from build123d import *

# Parameters (mm, degrees)
F1_DEPTH = 19.05
F2_R     = 1.5
F3_DEPTH = 12.7
F4_R     = 2.5
F5_DEPTH = 12.7


with BuildPart() as f1:
    # F0 (on Front) → F1 (new body)
    with BuildSketch(Plane.XZ):
        with BuildLine():
            Line((-43.747465, 0), (6.252535, 0))
            Line((6.252535, 0), (6.252535, 1.900001))
            Line((6.252535, 1.900001), (-43.747465, 1.900001))
            ThreePointArc((-43.747465, 1.900001), (-46.057163, 3.443292), (-45.515231, 6.167766))
            Line((-45.515231, 6.167766), (-27.837562, 23.845436))
            Line((-27.837562, 23.845436), (-29.181065, 25.188939))
            Line((-29.181065, 25.188939), (-46.858735, 7.51127))
            ThreePointArc((-46.858735, 7.51127), (-47.812535, 2.716193), (-43.747465, 0))
        make_face()
    extrude(amount=-F1_DEPTH)

    # F2 (on face) → F3 (cut)
    with BuildSketch(Plane(origin=(-27.185002, 0, 27.185002), x_dir=(0, -1, 0), z_dir=(-0.707107, 0, 0.707107))):
        with Locations((-7.5, -10.322859)):
            Circle(F2_R)
        with Locations((-11.55, -10.322859)):
            Circle(F2_R)
    extrude(amount=-F3_DEPTH, mode=Mode.SUBTRACT)

    # F4 (on face) → F5 (cut)
    with BuildSketch(Plane(origin=(0, 0, 0), x_dir=(1, 0, 0), z_dir=(0, 0, -1))):
        with BuildLine():
            Line((-5.372359, -7.282656), (-16.72876, -7.282656))
            ThreePointArc((-16.72876, -7.282656), (-18.690573, -10.030443), (-16.175304, -12.282656))
            Line((-16.175304, -12.282656), (-5.164585, -12.282656))
            ThreePointArc((-5.164585, -12.282656), (-3.70868, -9.717839), (-5.372359, -7.282656))
        make_face()
        with Locations((-25.747465, -9.375455)):
            Circle(F4_R)
    extrude(amount=-F5_DEPTH, mode=Mode.SUBTRACT)


solid = f1.part
Source: CAD feature listing. Evaluate the final solid. Frame: model axes, mm. A direction names the side the tool comes from. Round coordinates to 2 decimals unless told otherwise and drop trailing zeros. Loops run counter-clockwise (first coordinate to the right, second up) from the corner with the lowest first, then second, coordinate; pieces in that order, holes last. Notation, with made-up numbers: (-35.5, 62) - (-8.5, 62) arc R22 cw to (-8.5, 99) - close; hole circle Ø10 at (23, 74). An arc over 180 degrees is marked (long way). Write item = value, one per line. Start each with the question number.
(1) Section query D-D, the plane x = -42.5. Output: boundary loops of the cut face in (y, z).
(2) Ray query, line 1 along Z through (x, y) = (2.5, 5.25); line 2 along X through (y, z) = (10.5, 4.5); line 3 along Z through (x, y) = (-30.5, 3.5). Return the intervals inside material, ascending. Write a range as from..to.
(3) Pin query (flat end, axial travel): pin 1 (4 mm diameter, centred on y = 11.5, z = 14, fed in from +X); pin 2 (6 mm diameter, centred on y = 9.5, z = 15, fed in from -X); pin 3 (5 mm diameter, centred on y = 9, z = 10.5, fed in from +X). Return the tip coordinate at first contact, or that it passes through.
(4) Section query A-A, the plane x = -6. Output: boundary loops of the cut face in (y, z), plus the area to 3 significant figures.
(5) Pull-direction query (Z, two-part tool) for faces 1 (the face through (-3.707, 9.761, 0.937)), 2 (the face through (-46.041, 9.392, 3.405)), 3 (the face through (-19, 9, 0)); classes: +Z half, -Z half, draft (parallel to the pull), parting line (faces both ways), or undercut.
(6) Section query B-B, the plane y = 11.25. Output: boundary loops of the cut face in (x, z).
(7) Set-up query: faces 4 (the face through (-11, 12.283, 1)), 5 (the face through (-18, 7, 1.9)), 6 (the face through (-28.5, 9.39, 24.51)). Return all of +Z, -Z, +X, -X, +Y, -Y with unobstructed straight access to the full face (end or side cutting, diameter ignored); none if empty.
(8) Section query C-C, the plane y = 16.5. Output: boundary loops of the cut face in (x, z).
Conclusion:
q1.outline = (0, 0) - (19.05, 0) - (19.05, 1.9) - (0, 1.9) - close; (0, 9.18) - (19.05, 9.18) - (19.05, 11.87) - (0, 11.87) - close
q2.line_1 = 0..1.9
q2.line_2 = -48.15..-46.25
q2.line_3 = 0..1.9, 21.18..23.87
q3.pin_1 = -35.68
q3.pin_2 = -42.37
q3.pin_3 = -38.68
q4.outline = (0, 0) - (7.28, 0) - (7.28, 1.9) - (0, 1.9) - close; (12.28, 0) - (19.05, 0) - (19.05, 1.9) - (12.28, 1.9) - close
q4.area = 26.7 mm2
q5.face_1 = draft
q5.face_2 = undercut
q5.face_3 = -Z half
q6.outline = (-46.86, 7.51) arc R4.4 ccw to (-43.75, 0) - (-27.4, 0) - (-27.4, 1.9) - (-43.75, 1.9) arc R2.5 cw to (-45.52, 6.17) - (-34.18, 17.5) - (-35.52, 18.85) - close; (-33.45, 20.92) - (-32.1, 19.58) - (-27.84, 23.85) - (-29.18, 25.19) - close; (-24.09, 0) - (-18.21, 0) - (-18.21, 1.9) - (-24.09, 1.9) - close; (-4.09, 0) - (6.25, 0) - (6.25, 1.9) - (-4.09, 1.9) - close
q7.face_4 = +Z, -Z
q7.face_5 = +X, +Y, -Y
q7.face_6 = +Z, +X, +Y, -Y
q8.outline = (-46.86, 7.51) arc R4.4 ccw to (-43.75, 0) - (6.25, 0) - (6.25, 1.9) - (-43.75, 1.9) arc R2.5 cw to (-45.52, 6.17) - (-27.84, 23.85) - (-29.18, 25.19) - close
